from build123d import *

# Parameters (mm, degrees)
SKETCH_1_R      = 1
EXTRUDE_1_DEPTH = 2


with BuildPart() as part:
    # 草圖1 → 填料-伸長1 (new body)
    with BuildSketch(Plane.XY):
        with BuildLine():
            Line((-13.655498481, 25.979826384), (-13.655498481, 26.979826384))
            Line((-13.655498481, 26.979826384), (-12.655498481, 26.979826384))
            Line((-12.655498481, 26.979826384), (-1.655498481, 26.979826384))
            ThreePointArc((-1.655498481, 26.979826384), (-0.655498481, 25.979826384), (0.344501519, 26.979826384))
            Line((0.344501519, 26.979826384), (0.344501519, 28.979826384))
            Line((0.344501519, 28.979826384), (4.344501519, 28.979826384))
            Line((4.344501519, 28.979826384), (4.344501519, 26.979826384))
            ThreePointArc((4.344501519, 26.979826384), (5.344501519, 25.979826384), (6.344501519, 26.979826384))
            Line((6.344501519, 26.979826384), (10.344501519, 26.979826384))
            ThreePointArc((10.344501519, 26.979826384), (11.344501519, 25.979826384), (12.344501519, 26.979826384))
            Line((12.344501519, 26.979826384), (12.344501519, 28.979826384))
            Line((12.344501519, 28.979826384), (16.344501519, 28.979826384))
            Line((16.344501519, 28.979826384), (16.344501519, 26.979826384))
            ThreePointArc((16.344501519, 26.979826384), (17.344501519, 25.979826384), (18.344501519, 26.979826384))
            Line((18.344501519, 26.979826384), (29.344501519, 26.979826384))
            Line((29.344501519, 26.979826384), (30.344501519, 26.979826384))
            Line((30.344501519, 26.979826384), (30.344501519, 25.979826384))
            Line((30.344501519, 25.979826384), (30.344501519, -26.620173616))
            Line((30.344501519, -26.620173616), (29.344501519, -26.620173616))
            Line((29.344501519, -26.620173616), (18.344501519, -26.620173616))
            ThreePointArc((18.344501519, -26.620173616), (17.344501519, -25.620173616), (16.344501519, -26.620173616))
            Line((16.344501519, -26.620173616), (16.344501519, -28.620173616))
            Line((16.344501519, -28.620173616), (12.344501519, -28.620173616))
            Line((12.344501519, -28.620173616), (12.344501519, -26.620173616))
            ThreePointArc((12.344501519, -26.620173616), (11.344501519, -25.620173616), (10.344501519, -26.620173616))
            Line((10.344501519, -26.620173616), (6.344501519, -26.620173616))
            ThreePointArc((6.344501519, -26.620173616), (5.344501519, -25.620173616), (4.344501519, -26.620173616))
            Line((4.344501519, -26.620173616), (4.344501519, -28.620173616))
            Line((4.344501519, -28.620173616), (0.344501519, -28.620173616))
            Line((0.344501519, -28.620173616), (0.344501519, -26.620173616))
            ThreePointArc((0.344501519, -26.620173616), (-0.655498481, -25.620173616), (-1.655498481, -26.620173616))
            Line((-1.655498481, -26.620173616), (-12.655498481, -26.620173616))
            Line((-12.655498481, -26.620173616), (-13.655498481, -26.620173616))
            Line((-13.655498481, -26.620173616), (-13.655498481, 25.979826384))
        make_face()
        with Locations((14.344501519, 24.979826384)):
            Circle(SKETCH_1_R, mode=Mode.SUBTRACT)
        with Locations((2.344501519, -24.620173616)):
            Circle(SKETCH_1_R, mode=Mode.SUBTRACT)
        with Locations((14.344501519, -24.620173616)):
            Circle(SKETCH_1_R, mode=Mode.SUBTRACT)
        with Locations((2.344501519, 24.979826384)):
            Circle(SKETCH_1_R, mode=Mode.SUBTRACT)
    extrude(amount=EXTRUDE_1_DEPTH)


solid = part.part
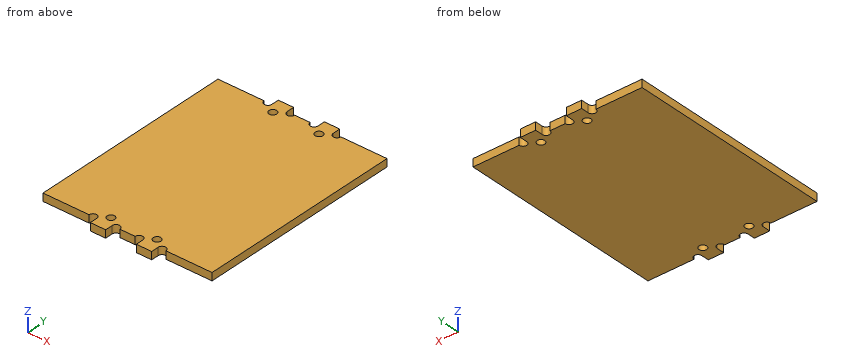
Part model, mm, in its own coordinate system. Round coordinates to 2 decimals unless told otherwise and drop trailing zeros. Write each loop counter-clockwise with the first axis right and the second up, starting at its lowest first coordinate (ties: lowest second). Pieces come first, ordered by that corner, then holes. Notation, with made-up numbers: M 31,-10.75 L 59,-10.75 A23 ccw 59,9.25 Z; hole C -0.5,73 d7. An arc over 180 degrees is marked long. Return JSON: item names as keys, results as strings. Group by question number.
(1) Saw through at B-B on x = -9. Write the cut outline in (y, z).
(2) Saw through at A-A on z = 1.3. Count the separate pieces of the cut face and the enclosed holes in it, then the cut area to 3 significant figures.
(3) Drill centre lines: probe 1 along X at (y, z) = (-24.5, 0.95); probe 2 along X at (y, z) = (25, 1.55); probe 3 along Y at (x, z) = (15, 1.1). Where is each one in solid material? Low to high.
(4) Pin check, flat tips, straight feed: pin 1 Ø1 at (y, z) = (-27.5, 1.5) entering from +X; pin 2 Ø1 at (y, z) = (28, 0.5) entering from -X. Stop position of each tip, or through.
Returned:
{
 "1": {"outline": "M -26.62,0 L 26.98,0 L 26.98,2 L -26.62,2 Z"},
 "2": {"separate pieces": "1", "enclosed holes": "4", "area": "2,370 mm²"},
 "3": {"probe 1": "-13.66 to 1.35, 3.34 to 13.35, 15.34 to 30.34", "probe 2": "-13.66 to 1.34, 3.34 to 13.34, 15.34 to 30.34", "probe 3": "-28.62 to -25.38, -23.86 to 24.22, 25.74 to 28.98"},
 "4": {"pin 1": "x = 16.34", "pin 2": "x = 0.34"}
}
